from build123d import *

# Parameters (mm, degrees)
BOSS_EXTRUDE1_DEPTH = 150
CUT_EXTRUDE1_DEPTH  = 101


with BuildPart() as part:
    # Sketch1 → Boss-Extrude1 (new body)
    with BuildSketch(Plane(origin=(0, 0, 0), x_dir=(0, 0, -1), z_dir=(1, 0, 0))):
        Polygon((0, 0), (-94, -54.270925304), (-100, -54.270925304), (0, 3.464101615), align=None)
    extrude(amount=BOSS_EXTRUDE1_DEPTH)

    # Sketch2 → Cut-Extrude1 (cut, through all)
    with BuildSketch(Plane.XY):
        Polygon((102.5, 0), (102.5, -29), (47.5, -29), (47.5, 0), (47.5, 3.464101615), (102.5, 3.464101615), align=None)
    extrude(amount=CUT_EXTRUDE1_DEPTH, mode=Mode.SUBTRACT)


solid = part.part
The model under review builds one solid part; all positions refer to its coordinate system, in mm. A direction names the side the tool comes from. Round coordinates to 2 decimals unless told otherwise and drop trailing zeros. Order: outer loops, then holes, each group sorted by start corner. A loop starts at its lowest first (then second) coordinate and runs counter-clockwise, first axis right, second up. Notation, with made-up numbers: (23, -17.5) -> (45, -17.5) arc R24 ccw to (45, -6.5) -> close; hole circle Ø10 at (-9, -19.75). An arc over 180 degrees is marked (long way). Write item = value, one per line. Start each with the question number.
Item 1: Consider section B-B on y = -15. Write out the cut boundary in (x, z).
Item 2: Mouldability with a two-part tool opening along X and no side actions: class faces 1 (the face through (47.5, -14, 26)), 2 (the face through (0, -27, 50)), 3 (the face through (150, -27, 50)), 4 (the face through (126, 2, 0)) as released by +X, released by -X, zero draft, split by the parting line, or undercut.
Item 3: Consider section A-A on z = 38. Write out the cut boundary in (x, y), plus the area to 3 significant figures.
Item 4: For faces 5 (the face through (23, 2, 0)), 6 (the face through (75, -29, 53)), list the 3-axis set-ups (+Z, -Z, +X, -X, +Y, -Y) from which the entire face can be reached by the end or side of a thin tool; tool diameter is ignored.
Item 5: For line 1 along Z through (x, y) = (124.5, 0); line 2 along Y through (x, z) = (40, 94.5); line 3 along Y through (x, z) = (18, 19), list the stretches that pass through material, from the lowest coordinate up.
Item 6: Consider section D-D on z = 54. Write out the cut boundary in (x, y), plus the area to 3 significant figures.
Item 7: Clearance check with flat-ended pins moving along their axes: pin 1 Ø4 at (x, z) = (15, 13) entering from -Y; pin 2 Ø8 at (x, z) = (35.5, 57) entering from -Y; pin 3 Ø8 at (x, y) = (17.5, -30.5) entering from +Z. State where each tip first meets the part, or that it passes through.
Item 8: Consider section C-C on x = 88. Write out the cut boundary in (y, z), plus the area to 3 significant figures.
Conclusion:
q1.outline = (0, 25.98) -> (47.5, 25.98) -> (47.5, 31.98) -> (0, 31.98) -> close; (102.5, 25.98) -> (150, 25.98) -> (150, 31.98) -> (102.5, 31.98) -> close
q2.face_1 = undercut
q2.face_2 = released by -X
q2.face_3 = released by +X
q2.face_4 = zero draft
q3.outline = (0, -21.94) -> (47.5, -21.94) -> (47.5, -18.48) -> (0, -18.48) -> close; (102.5, -21.94) -> (150, -21.94) -> (150, -18.48) -> (102.5, -18.48) -> close
q3.area = 329 mm2
q4.face_5 = -Z, +X, -X, +Y, -Y
q4.face_6 = +Z, -Z, +Y
q5.line_1 = 0 to 6
q5.line_2 = -54.27 to -51.1
q5.line_3 = -10.97 to -7.51
q6.outline = (0, -31.18) -> (150, -31.18) -> (150, -27.71) -> (102.5, -27.71) -> (102.5, -29) -> (47.5, -29) -> (47.5, -27.71) -> (0, -27.71) -> close
q6.area = 449 mm2
q7.pin_1 = -8.66
q7.pin_2 = -35.22
q7.pin_3 = 65.76
q8.outline = (-54.27, 94) -> (-29, 50.23) -> (-29, 56.23) -> (-54.27, 100) -> close
q8.area = 152 mm2
